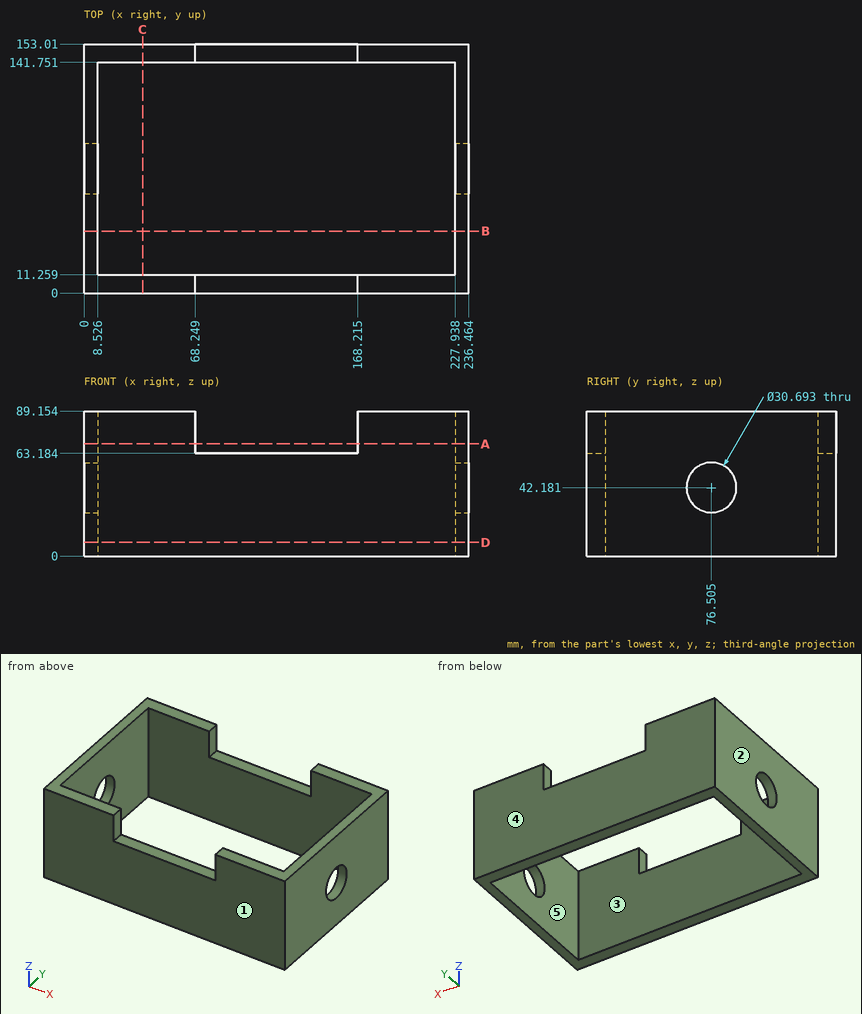
Input: dimensioned drawing with shaded views. Units: mm. Origin: part minimum x, y, z. A direction names the side the tool comes from. Round coordinates to 2 decimals unless told otherwise and drop trailing zeros. Order: outer loops, then holes, each group sorted by start corner. A loop starts at its lowest first (then second) coordinate and runs counter-clockwise, first axis right, second up. Notation, with made-up numbers: (64, -15.75) - (110, -15.75) arc R20 ccw to (110, 18.25) - close; hole circle Ø3 at (41, 21.5). An arc over 180 degrees is marked (long way). Answer as a JSON object with one key per item and string values. Group by question number.
(1) Cut plane B-B (y = 38). Return loops of the section in (x, z) (1 decimal), then the cut area to 3 significant figures.
(2) Draft query along X for the marked faces 1, 2 and 3. Return one class per face: released by +X, released by -X, zero draft, split by the parting line, or undercut.
(3) Cut plane A-A (z = 69). Return loops of the section in (x, y) (1 decimal), then the cut area to 3 significant figures.
(4) Cut plane D-D (z = 8.5). Return loops of the section in (x, y) (1 decimal).
(5) Reachability of the marked faces 4 and 5 from +Z, -Z, +X, -X, +Y, -Y: full face, straight path, thin tool, end or side. Return the list, or none.
(6) Material intervals for probe 1 along X at (y, z) = (48.5, 61) (1 decimal); probe 2 along Y at (x, z) = (226, 61), sorted ascending. Write a range as from..to.
(7) Cut plane C-C (x = 36). Return loops of the section in (y, z), then the cut area to 3 significant figures.
(8) Pin query (flat end, axial travel): P1, Ø5.5, axis at x = 120, y = 8, coming from the +Z side; P2, Ø8, axis at x = 89, z = 36.5, coming from the -Y side. Return the tip coordinate at first contact, or that it passes through.
Here are the results:
{
 "1": {"outline": "(0, 0) - (8.5, 0) - (8.5, 89.2) - (0, 89.2) - close; (227.9, 0) - (236.5, 0) - (236.5, 89.2) - (227.9, 89.2) - close", "area": "1,520 mm^2"},
 "2": {"face 1": "zero draft", "face 2": "released by -X", "face 3": "undercut"},
 "3": {"outline": "(0, 0) - (68.2, 0) - (68.2, 11.3) - (8.5, 11.3) - (8.5, 141.8) - (68.2, 141.8) - (68.2, 153) - (0, 153) - close; (168.2, 0) - (236.5, 0) - (236.5, 153) - (168.2, 153) - (168.2, 141.8) - (227.9, 141.8) - (227.9, 11.3) - (168.2, 11.3) - close", "area": "5,300 mm^2"},
 "4": {"outline": "(0, 0) - (236.5, 0) - (236.5, 153) - (0, 153) - close; hole (8.5, 11.3) - (227.9, 11.3) - (227.9, 141.8) - (8.5, 141.8) - close"},
 "5": {"face 4": "+Z, -Z, +X, -X, +Y", "face 5": "+Z, -Z"},
 "6": {"probe 1": "x = 0..8.5, 227.9..236.5", "probe 2": "y = 0..11.26, 141.75..153.01"},
 "7": {"outline": "(0, 0) - (11.26, 0) - (11.26, 89.15) - (0, 89.15) - close; (141.75, 0) - (153.01, 0) - (153.01, 89.15) - (141.75, 89.15) - close", "area": "2,010 mm^2"},
 "8": {"P1": "stops at z = 63.18", "P2": "stops at y = 0"}
}
